Input: dimensioned drawing with shaded views. Units: mm. Origin: part minimum x, y, z. A direction names the side the tool comes from. Give positions to 0.01 mm unless a question says otherwise; leave off trailing zeros. Write each loop counter-clockwise with the first axis right and the second up, starting at its lowest first coordinate (ties: lowest second). Pieces come first, ordered by that corner, then holes. Notation, with made-up numbers: (69, 69.25) - (110, 69.25) arc R21 cw to (110, 93.25) - close; hole circle Ø1 at (46.5, 87). An arc over 180 degrees is marked (long way). Answer as CSV lines item,"result".
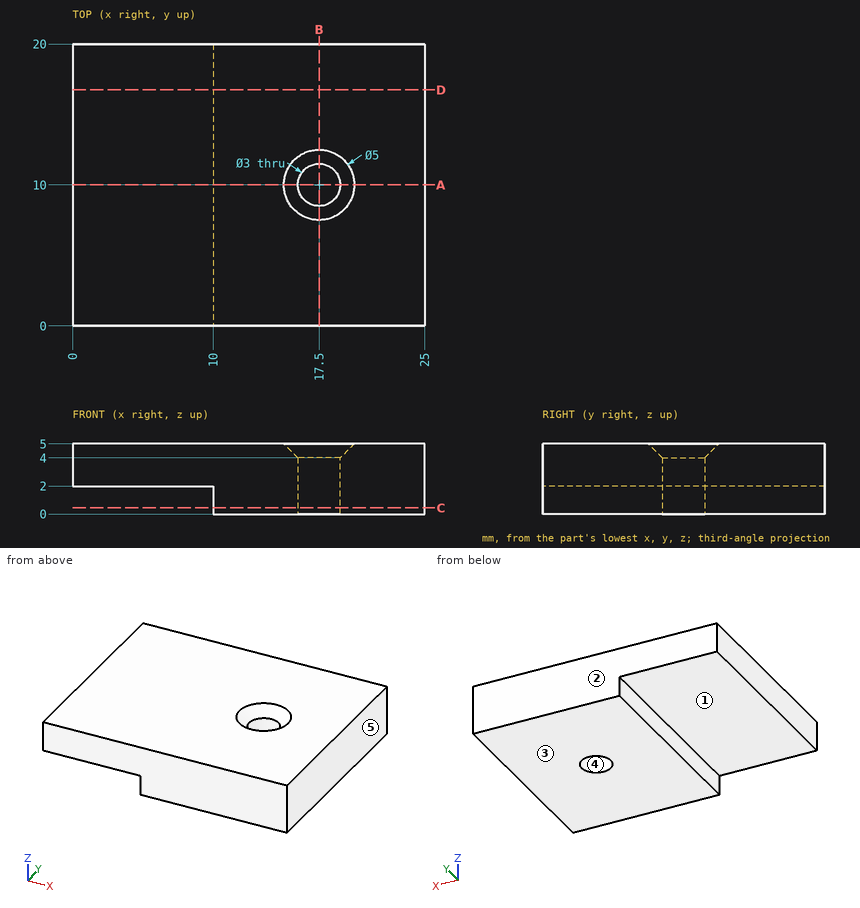
Item 1: Cut plane B-B on x = 17.5. Return the cut outline in (y, z).
The answers:
outline,"(0, 0) - (8.5, 0) - (8.5, 4) - (7.5, 5) - (0, 5) - close; (11.5, 0) - (20, 0) - (20, 5) - (12.5, 5) - (11.5, 4) - close"
Item 2: Contact query for flat-ended pins moving along their axis: pin 1 (3 mm diameter, centred on x = 3.5, y = 7.5, fed in from -Z); pin 2 (0.6 mm diameter, centred on y = 10, z = 1.5, fed in from -X). Output: stop coordinate, or through.
The answers:
pin 1,"z = 2"
pin 2,"x = 10"
Item 3: Ray query, line 1 (Y direction, x = 17.5, z = 3); line 2 (X direction, y = 10, z = 2.8); line 3 (X direction, y = 10, z = 1.9). Return the intervals inside material, ascending. Write a range as from..to.
The answers:
line 1,"0..8.5, 11.5..20"
line 2,"0..16, 19..25"
line 3,"10..16, 19..25"
Item 4: Mould query, pull axis X, two halves, no side actions, for the marked faces 3, 4 and 5. Classes: +X half, -X half, draft (parallel to the pull), parting line (faces both ways), or undercut.
The answers:
face 3,"draft"
face 4,"undercut"
face 5,"+X half"
Item 5: Cut plane C-C on z = 0.45. Return the cut outline in (x, y).
The answers:
outline,"(10, 0) - (25, 0) - (25, 20) - (10, 20) - close; hole circle Ø3 at (17.5, 10)"
Item 6: Cut plane A-A on y = 10. Return the cut outline in (x, z).
The answers:
outline,"(0, 2) - (10, 2) - (10, 0) - (16, 0) - (16, 4) - (15, 5) - (0, 5) - close; (19, 0) - (25, 0) - (25, 5) - (20, 5) - (19, 4) - close"
Item 7: Cut plane D-D on y = 16.75. Return the cut outline in (x, z), plus the area to 3 significant figures.
The answers:
outline,"(0, 2) - (10, 2) - (10, 0) - (25, 0) - (25, 5) - (0, 5) - close"
area,"105 mm²"
Item 8: Reachability of the marked faces 1 and 2 from +Z, -Z, +X, -X, +Y, -Y: full face, straight path, thin tool, end or side. Return the list, or none.
The answers:
face 1,"-Z, -X, +Y, -Y"
face 2,"+Z, -Z, +X, -X, +Y"
